Source: three-view drawing plus pictorial views. Frame: mm from the lowest corner of the part. A direction names the side the tool comes from. Give positions to 0.01 mm unless a question says otherwise; leave off trailing zeros. Loops run counter-clockwise (first coordinate to the right, second up) from the corner with the lowest first, then second, coordinate; pieces in that order, holes last. Notation, with made-up numbers: (26.5, 76.25) - (82.5, 76.25) arc R11 ccw to (82.5, 93.25) - close; hole circle Ø7 at (75.5, -22.5). An arc over 180 degrees is marked (long way). Answer as a JSON object with one key per item and string values.
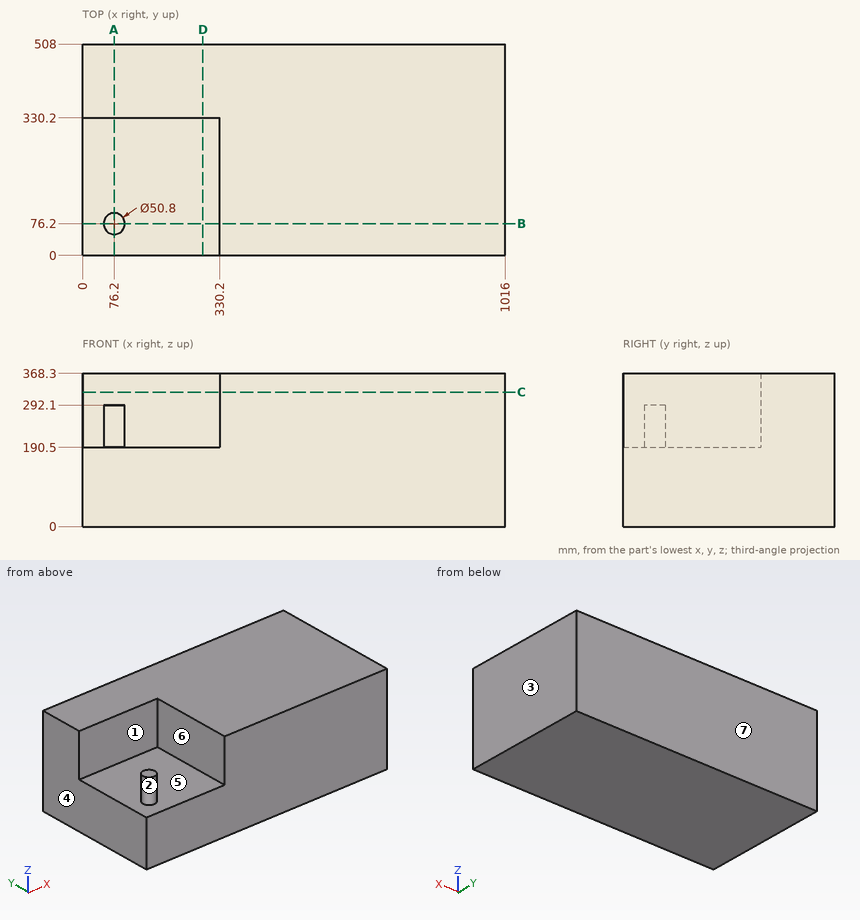
Item 1: Mould query, pull axis X, two halves, no side actions, for the marked faces 1, 2, 3 and 4. Classes: released by +X, released by -X, zero draft, split by the parting line, or undercut.
Geometry check:
{"face 1": "zero draft", "face 2": "undercut", "face 3": "released by +X", "face 4": "released by -X"}
Item 2: Cut plane A-A (x = 76.2). Return loops of the section in (y, z).
Geometry check:
{"outline": "(0, 0) - (508, 0) - (508, 368.3) - (330.2, 368.3) - (330.2, 190.5) - (101.6, 190.5) - (101.6, 292.1) - (50.8, 292.1) - (50.8, 190.5) - (0, 190.5) - close"}
Item 3: Cut plane C-C (z = 323). Return loops of the section in (x, y), then the cut area to 3 significant figures.
Geometry check:
{"outline": "(0, 330.2) - (330.2, 330.2) - (330.2, 0) - (1016, 0) - (1016, 508) - (0, 508) - close", "area": "407,000 mm2"}
Item 4: Access query for the marked faces 5, 6 and 7. Directions: +Z, -Z, +X, -X, +Y, -Y. A direction counts if a zero-diameter tool reaches every point of the face in a straight line with its end or side. Return the directions, or none.
Geometry check:
{"face 5": "+Z", "face 6": "+Z, -Y", "face 7": "+Z, -Z, +X, -X, +Y"}
Item 5: Cut plane D-D (x = 289.5). Return loops of the section in (y, z), then the cut area to 3 significant figures.
Geometry check:
{"outline": "(0, 0) - (508, 0) - (508, 368.3) - (330.2, 368.3) - (330.2, 190.5) - (0, 190.5) - close", "area": "128,000 mm2"}
Item 6: Material intervals for line 1 (Y direction, x = 49, z = 203.5); line 2 (X direction, y = 233, z = 219); line 3 (Z direction, x = 171.5, y = 170), sorted ascending. Write a range as [from, to].
Geometry check:
{"line 1": "y = [330.2, 508]", "line 2": "x = [330.2, 1016]", "line 3": "z = [0, 190.5]"}
Item 7: Cut plane B-B (y = 76.2). Return loops of the section in (x, z).
Geometry check:
{"outline": "(0, 0) - (1016, 0) - (1016, 368.3) - (330.2, 368.3) - (330.2, 190.5) - (101.6, 190.5) - (101.6, 292.1) - (50.8, 292.1) - (50.8, 190.5) - (0, 190.5) - close"}
